Autodesk Inventor part; units mm, degrees
ref_plane "YZ Plane" through (0, 0, 0) normal (1, 0, 0) x (0, 1, 0)
ref_plane "XZ Plane" through (0, 0, 0) normal (0, 1, 0) x (-1, 0, 0)
ref_plane "XY Plane" through (0, 0, 0) normal (0, 0, 1) x (1, 0, 0)
sketch "Sketch1" plane through (0, 0, 0) normal (1, 0, 0) x (0, 1, 0)
  line L0 (-29.5376, 40.3427) -> (-38, 55)
  circle A0 centre (0, 0) radius 50 construction
  line L1 (-38, 55) -> (-38.0101, 58)
  line L2 (-38.0101, 58) -> (-48.0101, 58)
  line L3 (-48.0101, 58) -> (-48, 55)
  line L4 (-58, 35) -> (-64, 35)
  line L5 (-64, 35) -> (-64, 45)
  line L6 (-64, 45) -> (-58, 45)
  arc A1 (-42.0654, 27.0278) -> (-29.5376, 40.3427) centre (0, 0) ccw construction
  line L7 (-58, 55) -> (-58, 45)
  line L8 (-38, 55) -> (-38, 55)
  line L9 (-48, 55) -> (-58, 55)
  line L10 (-58, 55) -> (-36.8235, 33.8235) construction
  line L11 (-50, 0) -> (-57.2434, 0)
  line L12 (-57.2434, 0) -> (-64, 0)
  line L13 (-64, 0) -> (-64, 10)
  line L14 (-64, 10) -> (-58, 10)
  line L15 (-58, 35) -> (-58, 10)
  arc A2 (-29.5376, 40.3427) -> (-50, 0) centre (0, 0) ccw
  point P0 (-30.8961, 39.312)
  dimension "d6" = 50
  dimension "d8" = 10
  dimension "d10" = 3
  dimension "d11" = 10
  dimension "d12" = 6
  dimension "d17" = 120
  dimension "d18" = 10
  dimension "d19" = 5
  dimension "d21" = 10
  dimension "d23" = 45
  dimension "d25" = 15
  dimension "d26" = 0
  dimension "d30" = 10
  dimension "d31" = 6
  dimension "d32" = 25
  dimension "d38" = 58
extrude "Extrusion2" add sketch "Sketch1" along normal blind 6
fillet "Fillet3" radius 5 2 edges at (3, -29.5376, 40.3427) (3, -50, 0)
sketch "Sketch2" plane through (6, 0, 0) normal (1, 0, 0) x (0, 0, -1)
  arc A0 (-41.7758, -37.2932) -> (-20.7846, -52) centre (0, 0) ccw
  line L0 (-20.7846, -52) -> (-49, -52)
  line L1 (-49, -52) -> (-49, -41.4641)
  line L2 (-49, -41.4641) -> (-41.7758, -37.2932)
  line L3 (-44.0661, -31.6873) -> (-55, -38)
  line L4 (-55, -48) -> (-55, -58)
  line L5 (-55, -58) -> (-45, -58)
  dimension "d42" = 6
  dimension "d43" = 6
  dimension "d44" = 6
  dimension "d45" = 56
extrude "Extrusion3" cut sketch "Sketch2" against normal through all
fillet "Fillet4" radius 1 1 edges at (3, -52, 20.7846)
fillet "Fillet5" radius 2 3 edges at (3, -52, 49) (3, -41.4641, 49) (3, -37.2932, 41.7758)
properties part number "HarnessPusher27021014"
Input: part model. Units: mm. Frame: model coordinates. A direction names the side the tool comes from. Round coordinates to 2 decimals unless told otherwise and drop trailing zeros. Write each loop counter-clockwise with the first axis right and the second up, starting at its lowest first coordinate (ties: lowest second). Pieces come first, ordered by that corner, then holes. Notation, with made-up numbers: (40.5, -31) -> (68.5, -31) arc R23 cw to (68.5, 8) -> close; hole circle Ø2 at (1, 86). An arc over 180 degrees is marked (long way). Answer as CSV lines item,"result".
1. Reachability of faces 4 (the flat face through (3, -58, 23)), 5 (the flat face through (3, -52, 36)), 6 (the flat face through (3, -53, 55)) from +Z, -Z, +X, -X, +Y, -Y: full face, straight path, thin tool, end or side. Return the list, or none.
Geometry says:
face 4,"+X, -X, -Y"
face 5,"+X, -X"
face 6,"+Z, +X, -X, -Y"
2. Mould query, pull axis Y, two halves, no side actions, for faces 1 (the flat face through (3, -58, 50)), 2 (the flat face through (3, -59, 0)), 3 (the cylindrical face through (2.958, -37.845, 41.893)). Classes: +Y half, -Y half, draft (parallel to the pull), parting line (faces both ways), or undercut.
Geometry says:
face 1,"-Y half"
face 2,"draft"
face 3,"undercut"
3. Section B-B (x = 4.55). Return the cut outline in (y, z).
Geometry says:
outline,"(-64, 0) -> (-54.77, 0) arc R5 ccw to (-49.79, 4.55) arc R50 cw to (-32.74, 37.79) arc R5 ccw to (-31.69, 44.07) -> (-38, 55) -> (-38.01, 58) -> (-48.01, 58) -> (-48, 55) -> (-58, 55) -> (-58, 45) -> (-64, 45) -> (-64, 35) -> (-58, 35) -> (-58, 10) -> (-64, 10) -> close; hole (-52, 25.46) arc R1 ccw to (-50.11, 25.01) arc R56 cw to (-38.45, 40.71) arc R2 ccw to (-38.09, 43.16) -> (-40.89, 48) arc R2 ccw to (-42.62, 49) -> (-50, 49) arc R2 ccw to (-52, 47) -> close"
4. Ray query, L1, parallel to Z at x = 4.6, y = -62; L2, parallel to Y at x = 3.4, z = 33; L3, parallel to Y at x = 0.35, z = 39. Return the intervals inside material, ascending. Write a range as [from, to].
Geometry says:
L1,"z = [0, 10], [35, 45]"
L2,"y = [-58, -52], [-45.24, -37.56]"
L3,"y = [-64, -52], [-40.19, -31.73]"
5. Section C-C (z = 29.5). Return the cut outline in (x, y), plus the area to 3 significant figures.
Geometry says:
outline,"(0, -58) -> (6, -58) -> (6, -52) -> (0, -52) -> close; (0, -47.6) -> (6, -47.6) -> (6, -40.37) -> (0, -40.37) -> close"
area,"79.4 mm^2"
6. Section D-D (z = 15). Return the cut outline in (x, y), plus the area to 3 significant figures.
Geometry says:
outline,"(0, -58) -> (6, -58) -> (6, -47.7) -> (0, -47.7) -> close"
area,"61.8 mm^2"
7. Section A-A (y = -60). Return the cut outline in (x, z), plus the area to 3 significant figures.
Geometry says:
outline,"(0, 0) -> (6, 0) -> (6, 10) -> (0, 10) -> close; (0, 35) -> (6, 35) -> (6, 45) -> (0, 45) -> close"
area,"120 mm^2"
8. Contact query for flat-ended pins moving along their axis: P1, Ø1.8, axis at x = 3, y = -60, coming from the +Z side; P2, Ø1.8, axis at x = 4, z = 20, coming from the -Y side; P3, Ø1.5, axis at x = 2.5, y = -43.5, coming from the -Z side. Output: stop coordinate, or through.
Geometry says:
P1,"stops at z = 45"
P2,"stops at y = -58"
P3,"stops at z = 23.28"
